from build123d import *

# Parameters (mm, degrees)
SKETCH1_R               = 1.65
BOSS_EXTRUDE1_DEPTH     = 10
CUT_EXTRUDE1_DEPTH      = 19.574175621
CUT_EXTRUDE1_DEPTH_BACK = 19.574175621
SKETCH2_W               = 21
SKETCH2_H               = 11
SKETCH4_W               = 36
SKETCH4_H               = 14
SKETCH4_R               = 1.65
BOSS_EXTRUDE2_DEPTH     = 7
BOSS_EXTRUDE3_DEPTH     = 5
FILLET1_R               = 4


with BuildPart() as part:
    # Sketch1 → Boss-Extrude1 (new, symmetric)
    with BuildSketch(Plane.XY):
        with BuildLine():
            Line((0, 7), (14, 7))
            Line((14, 7), (14, -7))
            Line((14, -7), (0, -7))
            ThreePointArc((0, -7), (-7, 0), (0, 7))
        make_face()
        Circle(SKETCH1_R, mode=Mode.SUBTRACT)
    extrude(amount=BOSS_EXTRUDE1_DEPTH, both=True)

    # Sketch2 → Cut-Extrude1 (cut, two sides: drawn at the far end of the back side and taken through both)
    with BuildSketch(Plane(origin=(0, 0, 0), x_dir=(1, 0, 0), z_dir=(0, 1, 0)).offset(-CUT_EXTRUDE1_DEPTH_BACK)):
        with Locations((3.5, 0)):
            Rectangle(SKETCH2_W, SKETCH2_H)
    extrude(amount=CUT_EXTRUDE1_DEPTH + CUT_EXTRUDE1_DEPTH_BACK, mode=Mode.SUBTRACT)


with BuildPart() as cut_extrude1_piece_1:
    # of the separate pieces the step leaves, piece 1, a body of its own (cut_extrude1_pieces)
    add(part.part.solids().sort_by_distance((0, 7, -10))[0])



with BuildPart() as cut_extrude1_piece_2:
    # of the separate pieces the step leaves, piece 2, a body of its own (cut_extrude1_pieces)
    add(part.part.solids().sort_by_distance((0, 7, 5.5))[0])


with BuildPart() as cut_extrude1_piece_1_1:
    add(cut_extrude1_piece_1.part)

    add(cut_extrude1_piece_2.part)  # Boss-Extrude2 merges Cut-Extrude1 piece 2
    # Sketch4 → Boss-Extrude2 (add)
    with BuildSketch(Plane(origin=(14, 0, 0), x_dir=(0, 0, -1), z_dir=(1, 0, 0))):
        Rectangle(SKETCH4_W, SKETCH4_H)
        with Locations((14, 0)):
            Circle(SKETCH4_R, mode=Mode.SUBTRACT)
        with Locations((-14, 0)):
            Circle(SKETCH4_R, mode=Mode.SUBTRACT)
    extrude(amount=BOSS_EXTRUDE2_DEPTH)

    # Sketch5 → Boss-Extrude3 (add)
    # profile 1 of 2: a face of its own
    with BuildSketch(Plane.ZY.offset(-14)):
        with BuildLine():
            Line((10, 3), (10, -3))
            ThreePointArc((10, -3), (14, -5), (18, -3))
            Line((18, -3), (18, 3))
            ThreePointArc((18, 3), (14, 5), (10, 3))
        make_face()
        Polygon((12.340117976, -2.875), (15.659882024, -2.875), (17.319764048, 0), (15.659882024, 2.875), (12.340117976, 2.875), (10.680235952, 0), align=None, mode=Mode.SUBTRACT)
    # profile 2 of 2: a face of its own
    with BuildSketch(Plane.ZY.offset(-14)):
        with BuildLine():
            Line((-18, 3), (-18, -3))
            ThreePointArc((-18, -3), (-14, -5), (-10, -3))
            Line((-10, -3), (-10, 3))
            ThreePointArc((-10, 3), (-14, 5), (-18, 3))
        make_face()
        Polygon((-10.680235952, 0), (-12.340117976, -2.875), (-15.659882024, -2.875), (-17.319764048, 0), (-15.659882024, 2.875), (-12.340117976, 2.875), align=None, mode=Mode.SUBTRACT)
    extrude(amount=BOSS_EXTRUDE3_DEPTH)

    # Fillet1
    fillet1_edges = [cut_extrude1_piece_1_1.edges().sort_by_distance(p)[0] for p in [
        (17.5, 7, 18),
        (17.5, -7, 18),
        (17.5, 7, -18),
        (17.5, -7, -18),
    ]]
    fillet(fillet1_edges, radius=FILLET1_R)


solid = cut_extrude1_piece_1_1.part
Could you check a few things on this model? Use its own coordinates, in mm. A direction names the side the tool comes from. Give positions to 0.01 mm unless a question says otherwise; leave off trailing zeros. Order: outer loops, then holes, each group sorted by start corner. A loop starts at its lowest first (then second) coordinate and runs counter-clockwise, first axis right, second up. Notation, with made-up numbers: (47, -31) - (57, -31) arc R20 cw to (57, -10) - close; hole circle Ø10 at (-17, -30.5). An arc over 180 degrees is marked (long way). Return JSON: item names as keys, results as strings. Group by question number.
Q1. Will these pins go through, and if not, where does the flat tip stop? pin 1 Ø7 at (x, y) = (1, -0.5) entering from -Z; pin 2 Ø1.5 at (x, z) = (-4, -10.5) entering from -Y; pin 3 Ø3 at (y, z) = (-6, 13) entering from -X.
Q2. Suppose I cut it at C-C, the plane y = 3.5. Please give me the cut outline in (x, z).
Q3. Suppose I cut it at B-B, the plane z = 9.5. Please give me the cut outline in (x, y), and give its area (3 significant figures).
Q4. Please list where these lines run through material, in increasing order: line 1 along Z through (x, y) = (0, 3.5); line 2 along Y through (x, z) = (0, -6.4); line 3 along X through (y, z) = (0, -8.45). Write a range as [from, to].
Q5. Suppose I cut it at D-D, the plane z = 0. Please give me the cut outline in (x, y).
Q6. Thinking about a two-plate mould opening in X: for faces 1 (the face through (14, 0, 0)), 2 (the face through (-1.216, 1.115, 7.719)), 3 (the face through (11.54, 1.42, -16.5)), which applies, pulls with the +X half, pulls with the -X half, needs draft (parallel to the pull), parting line crosses it, or undercut?
Q7. Suppose I cut it at A-A, the plane x = 10.75. Please give me the cut outline in (y, z) (3 decimals), and give its area (3 significant figures).
Q8. Which directions (+Z, -Z, +X, -X, +Y, -Y) give clear straight access to the entire face, cutting with the end or side of a thin tool? Please do faces 4 (the face through (11.535, -1.458, 16.478)), 5 (the face through (3, 0, 5.5)), 6 (the face through (9, 1, 11)), 7 (the face through (15, -7, 0)), 8 (the face through (9, 1, -17)).
Resolved:
{
 "1": {"pin 1": "stops at z = -10", "pin 2": "stops at y = -6.1", "pin 3": "stops at x = 9"},
 "2": {"outline": "(-6.06, -10) - (14, -10) - (14, -10.43) - (9, -10.43) - (9, -17.57) - (14, -17.57) - (14, -17.97) - (21, -17.97) - (21, 17.97) - (14, 17.97) - (14, 17.57) - (9, 17.57) - (9, 10.43) - (14, 10.43) - (14, 10) - (-6.06, 10) - (-6.06, 5.5) - (14, 5.5) - (14, -5.5) - (-6.06, -5.5) - close"},
 "3": {"outline": "(0, -7) - (21, -7) - (21, 7) - (0, 7) arc R7 ccw to start; hole circle Ø3.3 at (0, 0)", "area": "362 mm2"},
 "4": {"line 1": "z = [-10, -5.5], [5.5, 10]", "line 2": "y = [-7, -1.65], [1.65, 7]", "line 3": "x = [-7, -1.65], [1.65, 21]"},
 "5": {"outline": "(14, -7) - (21, -7) - (21, 7) - (14, 7) - close"},
 "6": {"face 1": "pulls with the -X half", "face 2": "undercut", "face 3": "needs draft"},
 "7": {"outline": "(-7, -10) - (-3, -10) arc R5 ccw to (-3, -18) - (3, -18) arc R5 ccw to (3, -10) - (7, -10) - (7, -5.5) - (-7, -5.5) - close; (-7, 5.5) - (7, 5.5) - (7, 10) - (3, 10) arc R5 ccw to (3, 18) - (-3, 18) arc R5 ccw to (-3, 10) - (-7, 10) - close; hole (-2.875, -15.66) - (0, -17.32) - (2.875, -15.66) - (2.875, -12.34) - (0, -10.68) - (-2.875, -12.34) - close; hole (-2.875, 12.34) - (0, 10.68) - (2.875, 12.34) - (2.875, 15.66) - (0, 17.32) - (-2.875, 15.66) - close", "area": "209 mm2"},
 "8": {"face 4": "-X", "face 5": "-X, +Y, -Y", "face 6": "+Z, -X, +Y, -Y", "face 7": "+Z, -Z, +X, -X, -Y", "face 8": "-Z, -X, +Y, -Y"}
}
